For this review, take the finished solid that the model builds, in its own axes (mm). A direction names the side the tool comes from. Coordinates: 2 decimals unless noted, no trailing zeros. Loops run counter-clockwise (first coordinate to the right, second up) from the corner with the lowest first, then second, coordinate; pieces in that order, holes last. Notation, with made-up numbers: (-6, -3) -> (14, -3) arc R20 cw to (14, 8) -> close; hole circle Ø2 at (-36, 44.5). An arc over 180 degrees is marked (long way). One line per item, written item: value.
from build123d import *

# Parameters (mm, degrees)
CIRKEL_R                   = 17
CILINDER_DEPTH             = 20
CIRKEL_GAT_R               = 5.1
OPENING_DEPTH              = 10
GATEN_PATROON_COUNT        = 3
CIRKEL1_R                  = 13.5
OPENING_OPZET_DEPTH        = 3
CIRKEL2_R                  = 2
GAT_VERLOOPSTUK_DEPTH      = 8
CIRKEL3_R                  = 3
GAT_VERLOOPSTUK_RAND_DEPTH = 2


with BuildPart() as part:
    # cirkel → cilinder (new body)
    with BuildSketch(Plane(origin=(0, 0, 0), x_dir=(1, 0, 0), z_dir=(0, 1, 0))):
        with Locations(Location((0, 0, 0), (0, 0, 270))):
            Circle(CIRKEL_R)
    extrude(amount=CILINDER_DEPTH)

    # boog → bol (revolve)
    with BuildSketch(Plane.XY):
        with BuildLine():
            Line((0, 20), (0, 37))
            ThreePointArc((0, 37), (-12.02081528, 32.02081528), (-17, 20))
            Line((-17, 20), (0, 20))
        make_face()
    revolve(axis=Axis((0, 20, 0), (0, 1, 0)))

    # cirkel_gat → opening (cut)
    with BuildSketch(Plane.XY.offset(17)):
        with Locations((0, 10)):
            Circle(CIRKEL_GAT_R)
    opening = extrude(amount=-OPENING_DEPTH, mode=Mode.SUBTRACT)

    # gaten_patroon: opening ×3 about axis
    gaten_patroon_axis = Axis((0, 0, 0), (0, 1, 0))
    for i in range(1, GATEN_PATROON_COUNT):
        add(opening.rotate(gaten_patroon_axis, i * 360 / GATEN_PATROON_COUNT), mode=Mode.SUBTRACT)

    # cirkel1 → opening_opzet (cut)
    with BuildSketch(Plane(origin=(0, 0, 0), x_dir=(-1, 0, 0), z_dir=(0, -1, 0))):
        with Locations(Location((0, 0, 0), (0, 0, 90))):
            Circle(CIRKEL1_R)
    extrude(amount=-OPENING_OPZET_DEPTH, mode=Mode.SUBTRACT)

    # cirkel2 → gat_verloopstuk (cut)
    with BuildSketch(Plane(origin=(0, 3, 0), x_dir=(-1, 0, 0), z_dir=(0, -1, 0))):
        with Locations(Location((0, 0, 0), (0, 0, 90))):
            Circle(CIRKEL2_R)
    extrude(amount=-GAT_VERLOOPSTUK_DEPTH, mode=Mode.SUBTRACT)

    # cirkel3 → gat_verloopstuk_rand (cut)
    with BuildSketch(Plane.XZ.offset(-3)):
        with Locations(Location((0, 0, 0), (0, 0, 270))):
            Circle(CIRKEL3_R)
    extrude(amount=-GAT_VERLOOPSTUK_RAND_DEPTH, mode=Mode.SUBTRACT)


solid = part.part
1. To check wall thickness, follow probe 1 along X at (y, z) = (7, 0); probe 2 along X at (y, z) = (13, -3); probe 3 along Y at (x, z) = (-9.5, -10). State the ranges of each line that lie inside material, in increasing order. Write a range as from..to.
Return value:
probe 1: x = -17..-8.25, -8.08..-2, 2..8.08, 8.25..17
probe 2: x = -16.73..-13.44, -6.35..6.35, 13.44..16.73
probe 3: y = 0..6.73, 13.27..29.94
2. Insertion check: pin 1 Ø12 at (x, z) = (-3.5, -2.5) entering from -Y; pin 2 Ø2 at (x, y) = (7, 23) entering from -Z; pin 3 Ø11 at (x, y) = (-1, 9.5) entering from +Z; pin 4 Ø4 at (x, z) = (3, 10) entering from +Y. Each pin has a flat end and moves straight along its axis. Give the tip position at first contact, or say it passes through.
Return value:
pin 1: stops at y = 3
pin 2: stops at z = -15.66
pin 3: stops at z = 17
pin 4: stops at y = 34.76
3. Take a section at B-B, the plane y = 10. Give the boundary of the cut face in (x, z).
Return value:
outline: (-16.59, -3.69) -> (-8.61, 0.92) -> (-3.51, -7.92) -> (-11.49, -12.53) arc R17 ccw to (11.49, -12.53) -> (3.51, -7.92) -> (8.61, 0.92) -> (16.59, -3.69) arc R17 ccw to (5.1, 16.22) -> (5.1, 7) -> (-5.1, 7) -> (-5.1, 16.22) arc R17 ccw to start; hole circle Ø4 at (0, 0)
4. Take a section at D-D, the plane y = 28.5. Give the boundary of the cut face in (x, z).
Return value:
outline: circle Ø29.44 at (0, 0)
5. The part is to be moulded in two halves that separate along Y. For faces 5 (the flat face through (13, 0, 5)), 6 (the cylindrical face through (10.786, 15.057, -5.461)), 7 (the cylindrical face through (0.9, 3.99, -2.86)), say which applies: pulls with the +Y half, pulls with the -Y half, needs draft (parallel to the pull), parting line crosses it, or undercut.
Return value:
face 5: pulls with the -Y half
face 6: undercut
face 7: needs draft
6. For faces 1 (the cylindrical face through (-13.18, 1.48, 2.93)), 2 (the cylindrical face through (-1, 15, 12)), 3 (the cylindrical face through (16.855, 9.86, -2.213)), 4 (the flat face through (6.098, 10.071, -3.438)), list the 3-axis set-ups (+Z, -Z, +X, -X, +Y, -Y) from which the entire face can be reached by the end or side of a thin tool; tool diameter is ignored.
Return value:
face 1: -Y
face 2: +Z
face 3: +Y, -Y
face 4: none
7. Take a section at C-C, the plane z = 1.5. Give the boundary of the cut face in (x, y).
Return value:
outline: (-16.93, 0) -> (-13.42, 0) -> (-13.42, 3) -> (-2.6, 3) -> (-2.6, 5) -> (-1.32, 5) -> (-1.32, 11) -> (1.32, 11) -> (1.32, 5) -> (2.6, 5) -> (2.6, 3) -> (13.42, 3) -> (13.42, 0) -> (16.93, 0) -> (16.93, 20) arc R16.93 ccw to (-16.93, 20) -> close
8. Take a section at A-A, the plane x = 0. Give the boundary of the cut face in (y, z), and give its area (3 significant figures).
Return value:
outline: (0, -17) -> (20, -17) arc R17 ccw to (20, 17) -> (15.1, 17) -> (15.1, 7) -> (4.9, 7) -> (4.9, 17) -> (0, 17) -> (0, 13.5) -> (3, 13.5) -> (3, 3) -> (5, 3) -> (5, 2) -> (11, 2) -> (11, -2) -> (5, -2) -> (5, -3) -> (3, -3) -> (3, -13.5) -> (0, -13.5) -> close
area: 915 mm2
